from build123d import *

# Parameters (mm, degrees)
F0_R     = 75
F0_R_2   = 4.5
F0_R_3   = 45
F1_DEPTH = 8
F2_R     = 3
F3_R     = 3


with BuildPart() as f1:
    # F0 (on Front) → F1 (new body)
    with BuildSketch(Plane.XZ):
        Circle(F0_R)
        with Locations((-27.125, -46.981878)):
            Circle(F0_R_2, mode=Mode.SUBTRACT)
        with Locations((-62.998735, -0.399298)):
            Circle(F0_R_2, mode=Mode.SUBTRACT)
        with Locations((31.84517, -54.358856)):
            Circle(F0_R_2, mode=Mode.SUBTRACT)
        with Locations((-27.125, 46.981878)):
            Circle(F0_R_2, mode=Mode.SUBTRACT)
        Circle(F0_R_3, mode=Mode.SUBTRACT)
        with Locations((54.25, 0)):
            Circle(F0_R_2, mode=Mode.SUBTRACT)
        with Locations((31.153565, 54.758154)):
            Circle(F0_R_2, mode=Mode.SUBTRACT)
    extrude(amount=F1_DEPTH)

    # F2
    f2_edges = [f1.edges().sort_by_distance(p)[0] for p in [
        (-45, 0, 0),
    ]]
    fillet(f2_edges, radius=F2_R)

    # F3
    f3_edges = [f1.edges().sort_by_distance(p)[0] for p in [
        (-75, 0, 0),
    ]]
    fillet(f3_edges, radius=F3_R)


solid = f1.part
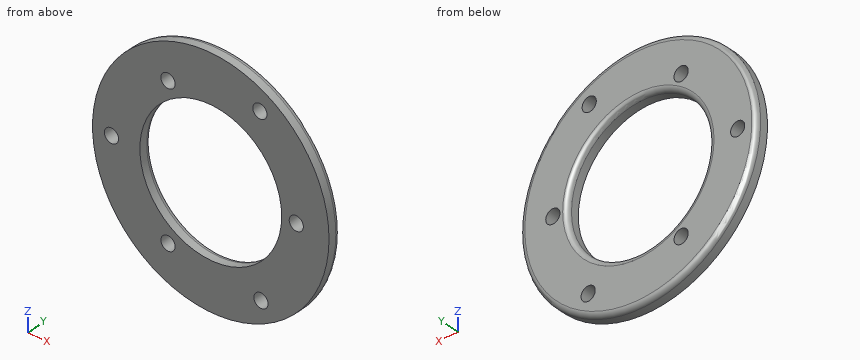
Input: part model. Units: mm. Frame: model coordinates. Give positions to 0.01 mm unless a question says otherwise; leave off trailing zeros. Order: outer loops, then holes, each group sorted by start corner. A loop starts at its lowest first (then second) coordinate and runs counter-clockwise, first axis right, second up. Notation, with made-up numbers: (53, 36) -> (111, 36) arc R28 ccw to (111, 55) -> close; hole circle Ø3 at (16.5, 84). An arc over 180 degrees is marked (long way). Use one line per item in the form item = value.
1) Section C-C, the plane x = -27. Count the separate pieces of the cut face and the enclosed holes in it, and give its area (3 significant figures).
Response values:
separate_pieces = 4
enclosed_holes = 0
area = 391 mm^2
2) Line query: probe 1 along Z at (x, y) = (-24.5, -7.25); probe 2 along Z at (x, y) = (28.5, -1.5); probe 3 along X at (y, z) = (-0.5, -3). Output: solid intervals per line, ascending.
Response values:
probe_1 = -70.89 to -50.64, -43.33 to -37.75, 37.75 to 43.33, 50.64 to 70.89
probe_2 = -68.94 to -57.37, -51.35 to -35.34, 35.34 to 51.12, 58.39 to 68.94
probe_3 = -73.6 to -66.67, -59.33 to -46.24, 46.24 to 50.9, 57.6 to 73.6
3) First-contact query: pin 1 Ø8 at (x, z) = (-63, -0.4) entering from +Y; pin 2 Ø1.5 at (y, z) = (-3, -55.5) entering from -X; pin 3 Ø2 at (x, y) = (14, -5.5) entering from +Z; pin 4 Ø4 at (x, y) = (44.5, -5) entering from +Z. Flat tips, straight axial feed; report the tip coordinate or a pass-through.
Response values:
pin_1 = through
pin_2 = -51.26
pin_3 = 73.86
pin_4 = 61.8
4) Section B-B, the plane y = -1.25. Return loops of the section in (x, z) (3 decimals), and give its area (3 significant figures).
Response values:
outline = circle Ø148.873 at (0, 0); hole circle Ø9 at (-62.999, -0.399); hole circle Ø91.127 at (0, 0); hole circle Ø9 at (-27.125, -46.982); hole circle Ø9 at (-27.125, 46.982); hole circle Ø9 at (31.154, 54.758); hole circle Ø9 at (31.845, -54.359); hole circle Ø9 at (54.25, 0)
area = 10,500 mm^2
5) Section A-A, the plane x = 0. Return loops of the section in (y, z).
Response values:
outline = (-8, -75) -> (-3, -75) arc R3 ccw to (0, -72) -> (0, -48) arc R3 ccw to (-3, -45) -> (-8, -45) -> close; (-8, 45) -> (-3, 45) arc R3 ccw to (0, 48) -> (0, 72) arc R3 ccw to (-3, 75) -> (-8, 75) -> close
